Autodesk Inventor part; units mm, degrees
ref_plane "YZ Plane" through (0, 0, 0) normal (1, 0, 0) x (0, 1, 0)
ref_plane "XZ Plane" through (0, 0, 0) normal (0, 1, 0) x (-1, 0, 0)
ref_plane "XY Plane" through (0, 0, 0) normal (0, 0, 1) x (1, 0, 0)
sketch "Boceto1" plane through (0, 0, 0) normal (0, 1, 0) x (-1, 0, 0)
  arc A0 (-45, 0) -> (45, 0) centre (0, 0) ccw
  line L0 (45, 0) -> (-45, 0)
  line L1 (25, -50) -> (-25, -50)
  line L2 (-25, -50) -> (-25, 50)
  line L3 (-25, 50) -> (25, 50)
  line L4 (25, 50) -> (25, -50)
  line L5 (25, -50) -> (-25, 50) construction
  line L6 (-25, -50) -> (25, 50) construction
  circle A1 centre (0, 50) radius 25
  point P0 (25, 0)
  point P1 (25, 50)
  point P2 (-25, 0)
  dimension "d0" = 90
  dimension "d1" = 50
  dimension "d2" = 100
extrude "Extrusión1" add sketch "Boceto1" along normal blind 10 contours L0 L2 A0 | L2 L0 L4 A0 | L2 A1 L4 L0 | L4 L0 A0 | A1 L3 | L3 A1
equation "\"d0\" = diametro_c"
equation "\"d1\" = ancho_p"
equation "\"d2\" = largo_p"
equation "\"d3\" = grueso"
equation "\"diametro_c\" = 90"
equation "\"grueso\" = 10"
equation "\"ancho_p\" = 50"
equation "\"largo_p\" = 100"
properties part number "Parte D" material "Madera (abedul)"
For this review, take the finished solid that the model builds, in its own axes (mm). A direction names the side the tool comes from. Coordinates: 2 decimals unless noted, no trailing zeros. Order: outer loops, then holes, each group sorted by start corner. A loop starts at its lowest first (then second) coordinate and runs counter-clockwise, first axis right, second up. Notation, with made-up numbers: (9.5, -35.5) - (46.5, -35.5) arc R15 ccw to (46.5, -11.5) - close; hole circle Ø11 at (57.5, -3). An arc over 180 degrees is marked (long way). Answer as CSV lines item,"result". Start each with the question number.
1) Insertion check: P1, Ø6, axis at y = 7, z = 4.5, coming from the -X side; P2, Ø3, axis at x = 38, y = 5, coming from the +Z side; P3, Ø2, axis at x = 9.5, y = 4, coming from the -Z side. Each pin has a flat end and moves straight along its axis. Give the tip position at first contact, or say it passes through.
2) To check wall thickness, follow line 1 along X through (y, z) = (6.25, 36); line 2 along Z through (x, y) = (1, 9.25); line 3 along X through (y, z) = (9.25, -39.5). State the ranges of each line that lie inside material, in increasing order. Write a range as [from, to].
3) Machinability: for faces 1 (the flat face through (1, 10, 16)), 2 (the flat face through (25, 5, 25)), 3 (the flat face through (-25, 5, 25)), which of the approach directions +Z, -Z, +X, -X, +Y, -Y give a long, thin tool a straight path to every point of the face, cutting with its end or side? Answer none if there is none.
4) Add section B-B (x = 27). State the section outline as (y, z) points, then the cut area to 3 significant figures.
5) Add section C-C (z = -29). State the section outline as (x, y) points, then the cut area to 3 significant figures.
6) Add section A-A (y = 2). State the section outline as (x, z) points, then the cut area to 3 significant figures.
Result:
1,P1,"x = -25"
1,P2,"z = 0"
1,P3,"z = -44.19"
2,line 1,"[-25, 25]"
2,line 2,"[-44.99, 74.98]"
2,line 3,"[-21.56, 21.56]"
3,face 1,"+Z, -Z, +X, -X, +Y"
3,face 2,"+Z, +X, +Y, -Y"
3,face 3,"+Z, -X, +Y, -Y"
4,outline,"(0, -36) - (10, -36) - (10, 0) - (0, 0) - close"
4,area,"360 mm^2"
5,outline,"(-34.41, 0) - (34.41, 0) - (34.41, 10) - (-34.41, 10) - close"
5,area,"688 mm^2"
6,outline,"(-45, 0) arc R45 ccw to (45, 0) - (25, 0) - (25, 50) arc R25 ccw to (-25, 50) - (-25, 0) - close"
6,area,"6,660 mm^2"
